```python
from build123d import *

# Parameters (mm, degrees)
TAP_DRILL_FOR_4_40_TAP1_REACH  = 195.495
TAP_DRILL_FOR_4_40_TAP1_BORE_R = 1.1303
CIRPATTERN2_COUNT              = 12


with BuildPart() as part:
    # Sketch2 → Revolve1 (revolve)
    with BuildSketch(Plane.XY, mode=Mode.PRIVATE) as revolve1_sk:
        with BuildLine():
            Line((0, 0), (56.388, 0))
            Line((56.388, 0), (56.388, 9.525))
            Line((56.388, 9.525), (40.513, 9.525))
            Line((40.513, 9.525), (40.513, 36.273710772))
            add(Edge.make_bspline(
                [(31.350017752, 77.94108456), (21.994739884, 61.495552558), (14.496239106, 54.512025578), (35.025537779, 38.606321532), (40.513, 36.273710772)],
                knots=[0, 0, 0, 0, 0.510148534, 0.739608491, 0.739608491, 0.739608491, 0.739608491], degree=3))
            Line((31.350017752, 77.94108456), (64.855703913, 135.974635332))
            ThreePointArc((64.855703913, 135.974635332), (64.855703913, 138.514635332), (62.655999387, 139.784635332))
            Line((62.655999387, 139.784635332), (55.88, 139.784635332))
            Line((55.88, 139.784635332), (6.35, 53.996158833))
            Line((6.35, 53.996158833), (6.35, 41.296158833))
            Line((6.35, 41.296158833), (21.780496632, 32.387357449))
            Line((21.780496632, 32.387357449), (21.780496632, 6.35))
            Line((21.780496632, 6.35), (0, 6.35))
            Line((0, 6.35), (0, 0))
        make_face()
    revolve(revolve1_sk.sketch.rotate(Axis((0, 6.35, 0), (0, -1, 0)), 90), axis=Axis((0, 6.35, 0), (0, -1, 0)))

    # Tap Drill for #4-40 Tap1 bore (on position points) → Tap Drill for #4-40 Tap1 (cut, up to next)
    with BuildSketch(Plane(origin=(0, 0, 51.6382), x_dir=(0, 0, -1), z_dir=(0, -1, 0)), mode=Mode.PRIVATE) as tap_drill_for_4_40_tap1_sk1:
        Circle(TAP_DRILL_FOR_4_40_TAP1_BORE_R)
    tap_drill_for_4_40_tap1_tool1 = extrude(tap_drill_for_4_40_tap1_sk1.sketch, amount=-TAP_DRILL_FOR_4_40_TAP1_REACH, mode=Mode.PRIVATE) & part.part
    tap_drill_for_4_40_tap1 = tap_drill_for_4_40_tap1_tool1.solids().sort_by_distance((0, 0, 51.6382))[0]
    add(tap_drill_for_4_40_tap1, mode=Mode.SUBTRACT)

    # CirPattern2: Tap Drill for #4-40 Tap1 ×12 about axis
    cirpattern2_axis = Axis((0, 0, 0), (0, 1, 0))
    for i in range(1, CIRPATTERN2_COUNT):
        add(tap_drill_for_4_40_tap1.rotate(cirpattern2_axis, i * 360 / CIRPATTERN2_COUNT), mode=Mode.SUBTRACT)


solid = part.part
```
The model under review builds one solid part; all positions refer to its coordinate system, in mm. A direction names the side the tool comes from. Round coordinates to 2 decimals unless told otherwise and drop trailing zeros. Write each loop counter-clockwise with the first axis right and the second up, starting at its lowest first coordinate (ties: lowest second). Pieces come first, ordered by that corner, then holes. Notation, with made-up numbers: (29, -33) - (33, -33) arc R16 cw to (33, -2) - close; hole circle Ø4 at (44.25, 36.5). An arc over 180 degrees is marked (long way). Use one line per item in the form item = value.
Q1. Insertion check: pin 1 Ø12 at (x, y) = (39.5, 29) entering from +Z; pin 2 Ø1.8 at (x, z) = (-25.82, 44.72) entering from +Y; pin 3 Ø2 at (y, z) = (77, -16) entering from -X. Each pin has a flat end and moves straight along its axis. Give the tip position at first contact, or say it passes through.
Answer key:
pin_1 = 22.78
pin_2 = 134
pin_3 = -27.22
Q2. Consider section A-A (y = 111.5). State the section outline as (x, z) points.
Answer key:
outline = circle Ø101.45 at (0, 0); hole circle Ø79.1 at (0, 0)
Q3. Tool access review of faces 5 (the cylindrical face through (50.026, 4.829, 26.02)), 6 (the cylindrical face through (3.86, 47.56, -5.04)), 7 (the flat face through (-1, 0, 1)), 8 (the cylindrical face through (-6.542, 19.186, 20.775)): name each direction out of +Z, -Z, +X, -X, +Y, -Y from which nothing blocks a thin tool from reaching the whole face with its end or side.
Answer key:
face_5 = -Y
face_6 = +Y
face_7 = +Z, -Z, +X, -X, -Y
face_8 = none
Q4. For line 1 (Y direction, x = 32, z = 27.5) (3 decimals); line 2 (X direction, y = 86.5, z = 9.5); line 3 (Z direction, x = -7, y = 100), list the stretches that pass through material, from the lowest coordinate up. Write a range as [from, to].
Answer key:
line_1 = [0, 9.525], [96.722, 116.078]
line_2 = [-35.03, -23.25], [23.25, 35.03]
line_3 = [-43.53, -32.16], [32.16, 43.53]
Q5. Draft analysis for pull direction X (two halves, no side actions). For faces 1 (the conical face through (6.49, 40.739, 3.376)), 2 (the flat face through (-38, 9.525, -17)), 3 (the conical face through (36.285, 88.02, -8.057)), 4 (the flat face through (0, 6.35, 0)), state which applies: +X half, -X half, draft (parallel to the pull), parting line (faces both ways), or undercut.
Answer key:
face_1 = undercut
face_2 = draft
face_3 = parting line
face_4 = undercut
